from build123d import *

# Parameters (mm, degrees)
SKETCH1_W          = 50
SKETCH1_H          = 50
SKETCH2_W          = 100
SKETCH2_H          = 100
SKETCH3_R          = 5
SKETCH6_R          = 5
SKETCH7_R          = 7.5
CUT_EXTRUDE1_DEPTH = 71.0000001


with BuildPart() as part:
    # Sketch1 → Loft1 section 0
    with BuildSketch(Plane(origin=(0, 0, 0), x_dir=(0, 0, -1), z_dir=(1, 0, 0))):
        Rectangle(SKETCH1_W, SKETCH1_H)
    # Sketch2 → Loft1 section 1
    with BuildSketch(Plane(origin=(-70, 0, 0), x_dir=(0, 0, -1), z_dir=(1, 0, 0))):
        Rectangle(SKETCH2_W, SKETCH2_H)
    loft()

    # Cut-Sweep2: sweep along a path in Sketch4
    with BuildLine(Plane(origin=(0, 0, 0), x_dir=(1, 0, 0), z_dir=(0, 1, 0))) as cut_sweep2_path:
        Line((0, 15), (-70, 40))
    # Sketch3 → Cut-Sweep2 (sweep, cut)
    with BuildSketch(Plane(origin=(0, 0, 0), x_dir=(0, 0, -1), z_dir=(1, 0, 0))):
        with Locations((15, 0)):
            Circle(SKETCH3_R)
    cut_sweep2 = sweep(path=cut_sweep2_path.line, mode=Mode.SUBTRACT)

    # Cut-Sweep3: sweep along a path in Sketch5
    with BuildLine(Plane.XY) as cut_sweep3_path:
        Line((0, 15), (-70, 40))
    # Sketch6 → Cut-Sweep3 (sweep, cut)
    with BuildSketch(Plane(origin=(0, 0, 0), x_dir=(0, 0, -1), z_dir=(1, 0, 0))):
        with Locations((0, 15)):
            Circle(SKETCH6_R)
    cut_sweep3 = sweep(path=cut_sweep3_path.line, mode=Mode.SUBTRACT)

    # Mirror1: Cut-Sweep2 across plane
    add(cut_sweep2.mirror(Plane.XY), mode=Mode.SUBTRACT)

    # Mirror2: Cut-Sweep3 across plane
    add(cut_sweep3.mirror(Plane.ZX), mode=Mode.SUBTRACT)

    # Sketch7 → Cut-Extrude1 (cut, through all)
    with BuildSketch(Plane(origin=(0, 0, 0), x_dir=(0, 0, -1), z_dir=(1, 0, 0))):
        Circle(SKETCH7_R)
    extrude(amount=-CUT_EXTRUDE1_DEPTH, mode=Mode.SUBTRACT)


solid = part.part
Verification items for the finished model (mm, model axes). Coordinates: 2 decimals unless noted, no trailing zeros. One line per item, written item: value. Start each with the question number.
Q1. Mould release check, pull along Y, two halves, no side actions. Record for faces 1 (the cylindrical face through (-34.51, 0.33, 7.493)), 2 (the flat face through (0, 6, 6)): pulls with the +Y half, pulls with the -Y half, needs draft (parallel to the pull), parting line crosses it, or undercut.
Q2. Thickness scan on L1, parallel to Y at x = -26, z = 0; L2, parallel to Y at x = -51.5, z = 0; L3, parallel to Z at x = -61.5, y = 4.5. Record the ranges inside material, lowest first. Write a range as from..to.
Q3. Cross-section at A-A on y = 0. State how many separate pieces and enclosed holes the cut face has, and give its area (3 significant figures).
Q4. Go/stop test with flat-tipped pins: P1, Ø12, axis at x = -30, z = -7.5, coming from the -Y side; P2, Ø6, axis at x = -53, z = -17, coming from the +Y side; P3, Ø4, axis at x = -59.5, y = -5.5, coming from the +Z side. Record where each tip stops, or that it passes through.
Checked values:
1. face 1: undercut
1. face 2: needs draft
2. L1: y = -34.29..-29.29, -19.29..-7.5, 7.5..19.29, 29.29..34.29
2. L2: y = -43.39..-38.39, -28.39..-7.5, 7.5..28.39, 38.39..43.39
2. L3: z = -46.96..-39.14, -34.78..-6, 6..34.78, 39.14..46.96
3. separate pieces: 4
3. enclosed holes: 0
3. area: 2,800 mm²
4. P1: stops at y = -37.86
4. P2: stops at y = 45
4. P3: stops at z = 46.96
